Verification items for the finished model (mm, model axes). A direction names the side the tool comes from. Give positions to 0.01 mm unless a question says otherwise; leave off trailing zeros. Order: outer loops, then holes, each group sorted by start corner. A loop starts at its lowest first (then second) coordinate and runs counter-clockwise, first axis right, second up. Notation, with made-up numbers: (63.25, 84.5) - (76.25, 84.5) arc R23 ccw to (76.25, 111.5) - close; hole circle Ø5 at (14.5, 14). An arc over 180 degrees is marked (long way). Answer as a JSON object with one key per item and string values.
```python
from build123d import *

# Parameters (mm, degrees)
ESQUISSE1_W             = 120.8
ESQUISSE1_H             = 8
BOSS_EXTRU_1_DEPTH      = 5
ESQUISSE2_W             = 10
ESQUISSE2_H             = 4
BOSS_EXTRU_2_DEPTH      = 10
ESQUISSE3_R             = 1.7
ENL_V_MAT_EXTRU_1_DEPTH = 10
ESQUISSE4_W             = 12
ESQUISSE4_H             = 20
BOSS_EXTRU_3_DEPTH      = 16
BOSS_EXTRU_3_DEPTH_BACK = 5
ESQUISSE5_R             = 4
ENL_V_MAT_EXTRU_2_DEPTH = 24
ESQUISSE6_R             = 1.7
ENL_V_MAT_EXTRU_3_DEPTH = 24


with BuildPart() as part:
    # Esquisse1 → Boss.-Extru.1 (new body)
    with BuildSketch(Plane.XY):
        Rectangle(ESQUISSE1_W, ESQUISSE1_H)
    extrude(amount=BOSS_EXTRU_1_DEPTH)

    # Esquisse2 → Boss.-Extru.2 (add)
    with BuildSketch(Plane(origin=(0, 0, 0), x_dir=(-1, 0, 0), z_dir=(0, 0, -1))):
        with Locations((24, -2)):
            Rectangle(ESQUISSE2_W, ESQUISSE2_H)
        with Locations((-24, 2)):
            Rectangle(ESQUISSE2_W, ESQUISSE2_H)
    extrude(amount=BOSS_EXTRU_2_DEPTH)

    # Esquisse3 → Enlèv. mat.-Extru.1 (cut)
    with BuildSketch(Plane(origin=(0, 4, 0), x_dir=(1, 0, 0), z_dir=(0, 1, 0))):
        with Locations((-24, 5)):
            Circle(ESQUISSE3_R)
        with Locations((24.35, 5)):
            Circle(ESQUISSE3_R)
    extrude(amount=-ENL_V_MAT_EXTRU_1_DEPTH, mode=Mode.SUBTRACT)

    # Esquisse4 → Boss.-Extru.3 (add, two sides)
    with BuildSketch(Plane(origin=(0, 0, 0), x_dir=(-1, 0, 0), z_dir=(0, 0, -1))) as boss_extru_3_sk:
        with Locations((54.4, 0)):
            Rectangle(ESQUISSE4_W, ESQUISSE4_H)
        with Locations((-54.4, 0)):
            Rectangle(ESQUISSE4_W, ESQUISSE4_H)
    extrude(amount=BOSS_EXTRU_3_DEPTH)
    extrude(boss_extru_3_sk.sketch, amount=-BOSS_EXTRU_3_DEPTH_BACK)

    # Esquisse5 → Enlèv. mat.-Extru.2 (cut)
    with BuildSketch(Plane(origin=(0, 0, -16), x_dir=(-1, 0, 0), z_dir=(0, 0, -1))):
        with Locations((54.4, 0)):
            Circle(ESQUISSE5_R)
        with Locations((-54.4, 0)):
            Circle(ESQUISSE5_R)
    extrude(amount=-ENL_V_MAT_EXTRU_2_DEPTH, mode=Mode.SUBTRACT)

    # Esquisse6 → Enlèv. mat.-Extru.3 (cut)
    with BuildSketch(Plane.XZ.offset(10)):
        with Locations((54.4, -9.479015636)):
            Circle(ESQUISSE6_R)
        with Locations((54.4, -1.479015636)):
            Circle(ESQUISSE6_R)
        with Locations((-54.4, -1.479015636)):
            Circle(ESQUISSE6_R)
        with Locations((-54.4, -9.479015636)):
            Circle(ESQUISSE6_R)
    extrude(amount=-ENL_V_MAT_EXTRU_3_DEPTH, mode=Mode.SUBTRACT)


solid = part.part
```
(1) Section check B-B (z = 3.5). Record the cut outline in (x, y).
Computed values:
{"outline": "(-60.4, -10) - (-48.4, -10) - (-48.4, -4) - (48.4, -4) - (48.4, -10) - (60.4, -10) - (60.4, 10) - (48.4, 10) - (48.4, 4) - (-48.4, 4) - (-48.4, 10) - (-60.4, 10) - close; hole circle Ø8 at (-54.4, 0); hole circle Ø8 at (54.4, 0)"}
(2) Gauge pin test, flat ends, axial feed: pin 1 Ø5 at (x, z) = (26, -5.5) entering from -Y; pin 2 Ø3 at (x, z) = (-24.5, -5) entering from +Y; pin 3 Ø3 at (x, y) = (-21.5, -2.5) entering from -Z. Record the tip position at first contact, or that the pin passes through.
Computed values:
{"pin 1": "stops at y = 0", "pin 2": "stops at y = 0", "pin 3": "stops at z = -10"}
(3) Section check A-A (x = -54.4). Record the cut outline in (y, z), then the cut area to 3 significant figures.
Computed values:
{"outline": "(-10, -16) - (-4, -16) - (-4, -11.18) - (-10, -11.18) - close; (-10, -7.78) - (-4, -7.78) - (-4, -3.18) - (-10, -3.18) - close; (-10, 0.22) - (-4, 0.22) - (-4, 5) - (-10, 5) - close; (4, -16) - (10, -16) - (10, -11.18) - (4, -11.18) - close; (4, -7.78) - (10, -7.78) - (10, -3.18) - (4, -3.18) - close; (4, 0.22) - (10, 0.22) - (10, 5) - (4, 5) - close", "area": "170 mm²"}
(4) Access from +Z, -Z, +X, -X, +Y, -Y to the whole of each face (thin tool, end or side, straight path). Record for faces 1 (the cylindrical face through (52.554, -3.549, -5.647)), 2 (the flat face through (-19, -2, -5)), 3 (the flat face through (22, 0, -5)).
Computed values:
{"face 1": "+Z, -Z", "face 2": "-Z, +Y, -Y", "face 3": "-Z, -Y"}
(5) Release check for a two-part mould opening along Z. For faces 4 (the flat face through (-29, -2, -5)), 5 (the flat face through (1, 0, 5)), 6 (the cylindrical face through (55.97, -6.86, -10.13)), 7 (the flat face through (-24, -2, -10)) record: pulls with the +Z half, pulls with the -Z half, needs draft (parallel to the pull), parting line crosses it, or undercut.
Computed values:
{"face 4": "needs draft", "face 5": "pulls with the +Z half", "face 6": "undercut", "face 7": "pulls with the -Z half"}
(6) Material ranges on line 1 along X through (y, z) = (6, -1.5); line 2 along Z through (x, y) = (54.4, -5.75); line 3 along X through (y, z) = (-6.25, -13), recorded low to high. Write a range as [from, to].
Computed values:
{"line 1": "x = [-60.4, -56.1], [-52.7, -48.4], [48.4, 52.7], [56.1, 60.4]", "line 2": "z = [-16, -11.18], [-7.78, -3.18], [0.22, 5]", "line 3": "x = [-60.4, -48.4], [48.4, 60.4]"}
(7) Section check C-C (y = -1.25). Record the cut outline in (x, z).
Computed values:
{"outline": "(-60.4, -16) - (-58.2, -16) - (-58.2, 5) - (-60.4, 5) - close; (-50.6, -16) - (-48.4, -16) - (-48.4, 0) - (-29, 0) - (-29, -10) - (-19, -10) - (-19, 0) - (48.4, 0) - (48.4, -16) - (50.6, -16) - (50.6, 5) - (-50.6, 5) - close; (58.2, -16) - (60.4, -16) - (60.4, 5) - (58.2, 5) - close; hole circle Ø3.4 at (-24, -5)"}
(8) Section check D-D (y = 7). Record the cut outline in (x, z).
Computed values:
{"outline": "(-60.4, -16) - (-48.4, -16) - (-48.4, 5) - (-60.4, 5) - close; (48.4, -16) - (60.4, -16) - (60.4, 5) - (48.4, 5) - close; hole circle Ø3.4 at (-54.4, -9.48); hole circle Ø3.4 at (-54.4, -1.48); hole circle Ø3.4 at (54.4, -9.48); hole circle Ø3.4 at (54.4, -1.48)"}
